from build123d import *

# Parameters (mm, degrees)
F3_W     = 104.4
F3_H     = 71.4
F6_DEPTH = 32.2
F4_W     = 101.2
F4_H     = 68.2
F7_DEPTH = 10
F5_W     = 98
F5_H     = 65
F8_DEPTH = 29
F9_R     = 3.2
F10_R    = 1.6


with BuildPart() as f6:
    # F3 (on Top) → F6 (new body)
    with BuildSketch(Plane.XY):
        Rectangle(F3_W, F3_H)
    extrude(amount=-F6_DEPTH)

    # F4 (on Top) → F7 (cut)
    with BuildSketch(Plane.XY):
        Rectangle(F4_W, F4_H)
    extrude(amount=-F7_DEPTH, mode=Mode.SUBTRACT)

    # F5 (on Top) → F8 (cut)
    with BuildSketch(Plane.XY):
        Rectangle(F5_W, F5_H)
    extrude(amount=-F8_DEPTH, mode=Mode.SUBTRACT)

    # F9
    f9_edges = [f6.edges().sort_by_distance(p)[0] for p in [
        (-52.2, -35.7, -16.1),
        (52.2, -35.7, -16.1),
        (52.2, 35.7, -16.1),
        (-52.2, 35.7, -16.1),
    ]]
    fillet(f9_edges, radius=F9_R)

    # F10
    f10_edges = [f6.edges().sort_by_distance(p)[0] for p in [
        (-50.6, 34.1, -5),
        (-50.6, -34.1, -5),
        (50.6, 34.1, -5),
        (50.6, -34.1, -5),
    ]]
    fillet(f10_edges, radius=F10_R)


solid = f6.part
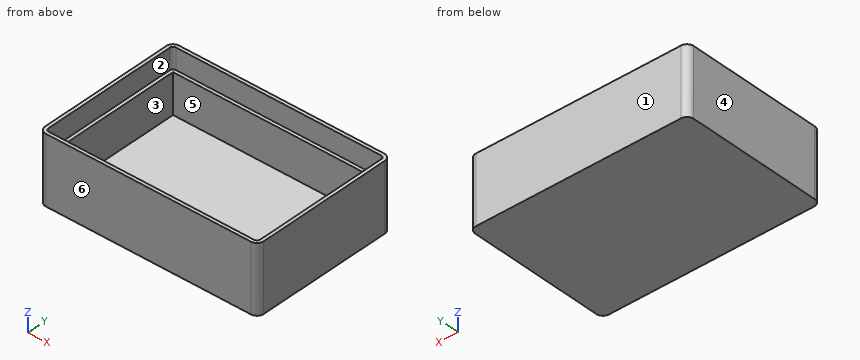
Verification items for the finished model (mm, model axes). Face numbers are marked on the shaded views. A direction names the side the tool comes from. Give positions to 0.01 mm unless a question says otherwise; leave off trailing zeros. Loops run counter-clockwise (first coordinate to the right, second up) from the corner with the lowest first, then second, coordinate; pieces in that order, holes last.
1. Cross-section at A-A on z = -15.5. Record the cut outline in (x, y), and give its area (3 significant figures).
Derived:
outline: (-52.2, -32.5) arc R3.2 ccw to (-49, -35.7) - (49, -35.7) arc R3.2 ccw to (52.2, -32.5) - (52.2, 32.5) arc R3.2 ccw to (49, 35.7) - (-49, 35.7) arc R3.2 ccw to (-52.2, 32.5) - close; hole (-49, -32.5) - (49, -32.5) - (49, 32.5) - (-49, 32.5) - close
area: 1,080 mm2
2. Cross-section at D-D on z = -6. Record the cut outline in (x, y), and give its area (3 significant figures).
Derived:
outline: (-52.2, -32.5) arc R3.2 ccw to (-49, -35.7) - (49, -35.7) arc R3.2 ccw to (52.2, -32.5) - (52.2, 32.5) arc R3.2 ccw to (49, 35.7) - (-49, 35.7) arc R3.2 ccw to (-52.2, 32.5) - close; hole (-50.6, -32.5) arc R1.6 ccw to (-49, -34.1) - (49, -34.1) arc R1.6 ccw to (50.6, -32.5) - (50.6, 32.5) arc R1.6 ccw to (49, 34.1) - (-49, 34.1) arc R1.6 ccw to (-50.6, 32.5) - close
area: 546 mm2
3. Material ranges on probe 1 along Y at (x, z) = (38, -22.5); probe 2 along Y at (x, z) = (-34, -9); probe 3 along X at (y, z) = (-31.5, -19.5), recorded low to high.
Derived:
probe 1: y = -35.7 to -32.5, 32.5 to 35.7
probe 2: y = -35.7 to -34.1, 34.1 to 35.7
probe 3: x = -52.2 to -49, 49 to 52.2
4. Release check for a two-part mould opening along X. For the marked faces 1, 2, 3 and 4 record: +X half, -X half, draft (parallel to the pull), parting line (faces both ways), or undercut.
Derived:
face 1: draft
face 2: undercut
face 3: undercut
face 4: -X half
5. Tool access check on the marked faces 5 and 6. Record the directions out of +Z, -Z, +X, -X, +Y, -Y that give a thin tool (end or side, any length) a straight path to the whole face; none if there is none.
Derived:
face 5: +Z
face 6: +Z, -Z, +X, -X, -Y
6. Go/stop test with a flat-tipped pin: P1, Ø12, axis at x = 27, y = 25, coming from the +Z side. Record where the tip stops, or that it passes through.
Derived:
P1: stops at z = -29
7. Cross-section at B-B on x = 33. Record the cut outline in (y, z), and give its area (3 significant figures).
Derived:
outline: (-35.7, -32.2) - (35.7, -32.2) - (35.7, 0) - (34.1, 0) - (34.1, -10) - (32.5, -10) - (32.5, -29) - (-32.5, -29) - (-32.5, -10) - (-34.1, -10) - (-34.1, 0) - (-35.7, 0) - close
area: 382 mm2
8. Cross-section at C-C on y = 5. Record the cut outline in (x, z), and give its area (3 significant figures).
Derived:
outline: (-52.2, -32.2) - (52.2, -32.2) - (52.2, 0) - (50.6, 0) - (50.6, -10) - (49, -10) - (49, -29) - (-49, -29) - (-49, -10) - (-50.6, -10) - (-50.6, 0) - (-52.2, 0) - close
area: 488 mm2
